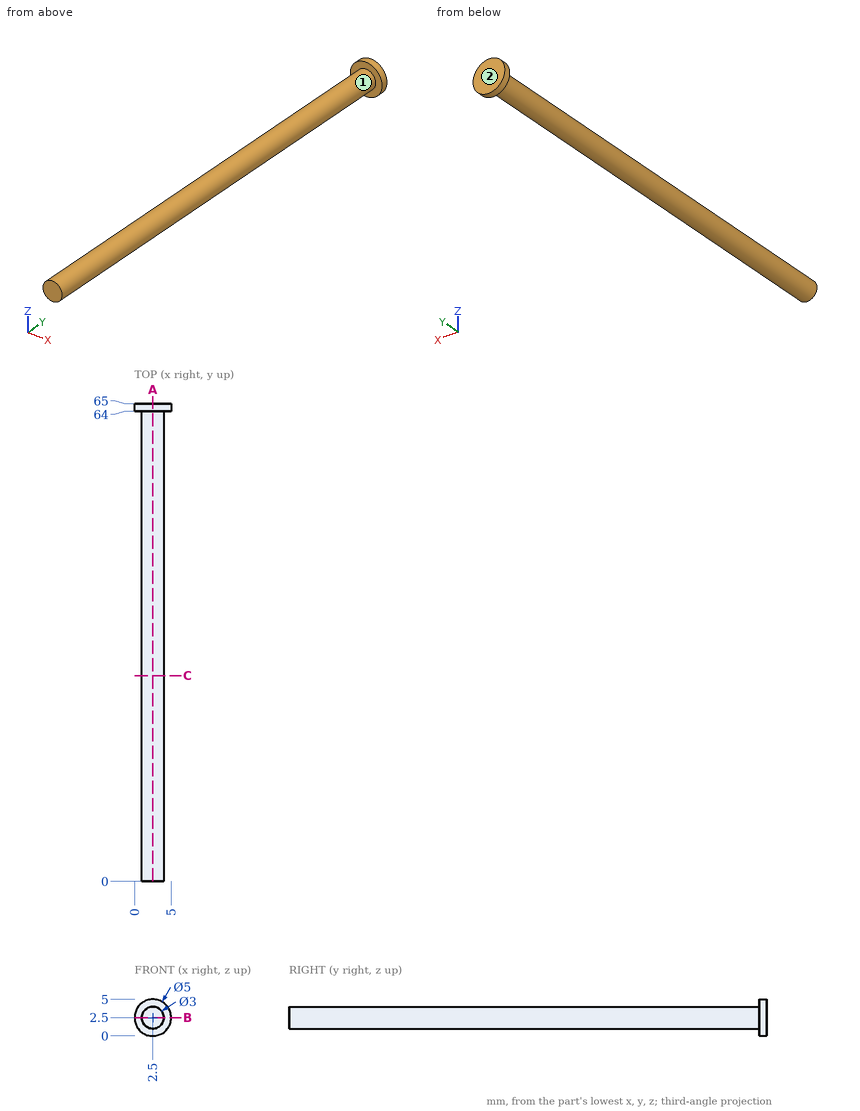
Here's the drawing with two shaded views (mm, measured from the low corner). I have some questions. A direction names the side the tool comes from. Give positions to 0.01 mm unless a question says otherwise; leave off trailing zeros. Loops run counter-clockwise (first coordinate to the right, second up) from the corner with the lowest first, then second, coordinate; pieces in that order, holes last. Notation, with made-up numbers: (60, 63.5) - (70, 63.5) arc R10 ccw to (70, 77.5) - close; hole circle Ø6 at (-38.75, -36). An arc over 180 degrees is marked (long way). Answer in a Markdown table with one row per item. Add a question column.
Q1. For pin 1 (1 mm diameter, centred on y = 14, z = 3.5, fed in from +X); pin 2 (3 mm diameter, centred on x = 0.5, y = 53, fed in from +Z), each with a flat end and sliding along its axis, tell me the tip position at first contact or that it passes through.
Q2. If we section it at C-C (y = 28): List the corners of the cut face in (x, z) for me, plus the area to 3 significant figures.
Q3. Which directions (+Z, -Z, +X, -X, +Y, -Y) give clear straight access to the entire face, cutting with the end or side of a thin tool? Please do the marked faces 1 and 2.
Q4. If we section it at A-A (x = 2.5): List the corners of the cut face in (y, z) for me.
Q5. If we section it at B-B (z = 2.5): List the corners of the cut face in (x, y) for me.
Q6. Please list where these lines run through material, in increasing order: L1, parallel to Y at x = 4, z = 2; L2, parallel to Z at x = 2.65, y = 19; L3, parallel to X at y = 60, z = 3. Write a range as from..to.
The answers:
| question | item | result |
|---|---|---|
| 1 | pin 1 | stops at x = 3.91 |
| 1 | pin 2 | stops at z = 3.91 |
| 2 | outline | circle Ø3 at (2.5, 2.5) |
| 2 | area | 7.07 mm^2 |
| 3 | face 1 | -Y |
| 3 | face 2 | +Z, -Z, +X, -X, +Y |
| 4 | outline | (0, 1) - (64, 1) - (64, 0) - (65, 0) - (65, 5) - (64, 5) - (64, 4) - (0, 4) - close |
| 5 | outline | (0, 64) - (1, 64) - (1, 0) - (4, 0) - (4, 64) - (5, 64) - (5, 65) - (0, 65) - close |
| 6 | L1 | y = 64..65 |
| 6 | L2 | z = 1.01..3.99 |
| 6 | L3 | x = 1.09..3.91 |
